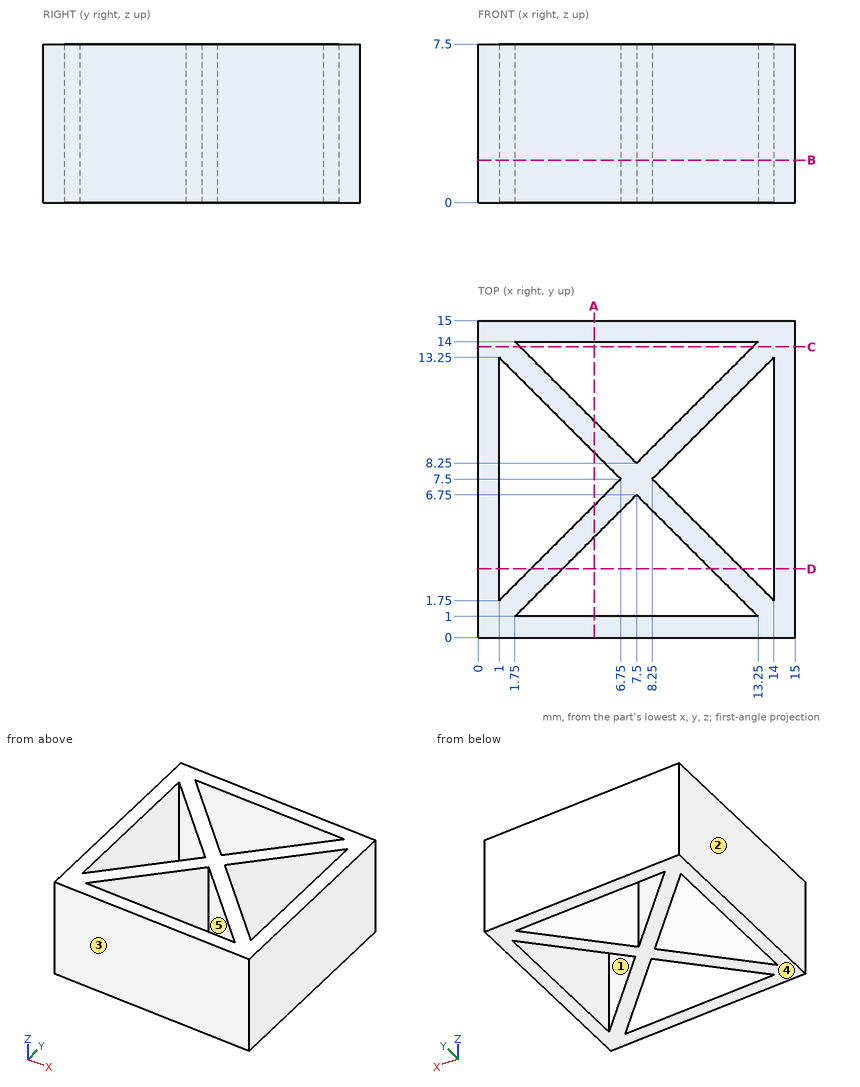
Answer from the drawing. Dimensions are ordinates in mm from the lowest x, y and z of the part. A direction names the side the tool comes from. Coordinates: 2 decimals unless noted, no trailing zeros. Order: outer loops, then holes, each group sorted by start corner. A loop starts at its lowest first (then second) coordinate and runs counter-clockwise, first axis right, second up. Notation, with made-up numbers: (-15.75, 52) - (5.25, 52) arc R14 cw to (5.25, 76) - close; hole circle Ø2 at (8.25, 61). An arc over 180 degrees is marked (long way). Use one line per item in the form item = value.
(1) Section D-D, the plane y = 3.25 is taken. Give the vertices of the cut face in (x, z).
Computed values:
outline = (0, 0) - (1, 0) - (1, 7.5) - (0, 7.5) - close; (2.5, 0) - (4, 0) - (4, 7.5) - (2.5, 7.5) - close; (11, 0) - (12.5, 0) - (12.5, 7.5) - (11, 7.5) - close; (14, 0) - (15, 0) - (15, 7.5) - (14, 7.5) - close
(2) Straight lines are drawn through the part: L1, parallel to Y at x = 10.75, z = 4.5; L2, parallel to X at y = 5.5, z = 2.5; L3, parallel to X at y = 8.5, z = 0.5. For each, find the intervals that lie inside material, in ascending order.
Computed values:
L1 = 0 to 1, 3.5 to 5, 10 to 11.5, 14 to 15
L2 = 0 to 1, 4.75 to 6.25, 8.75 to 10.25, 14 to 15
L3 = 0 to 1, 5.75 to 7.25, 7.75 to 9.25, 14 to 15
(3) For a pull along X with two mould halves and no side action, classify the marked faces 1, 2 and 3 as pulls with the +X half, pulls with the -X half, needs draft (parallel to the pull), parting line crosses it, or undercut.
Computed values:
face_1 = undercut
face_2 = pulls with the -X half
face_3 = needs draft
(4) Section C-C, the plane y = 13.75 is taken. Give the vertices of the cut face in (x, z), then the cut area to 3 significant figures.
Computed values:
outline = (0, 0) - (2, 0) - (2, 7.5) - (0, 7.5) - close; (13, 0) - (15, 0) - (15, 7.5) - (13, 7.5) - close
area = 30.0 mm²
(5) Section B-B, the plane z = 2 is taken. Give the vertices of the cut face in (x, y), then the cut area to 4 significant figures.
Computed values:
outline = (0, 0) - (15, 0) - (15, 15) - (0, 15) - close; hole (1, 1.75) - (6.75, 7.5) - (1, 13.25) - close; hole (1.75, 1) - (13.25, 1) - (7.5, 6.75) - close; hole (1.75, 14) - (7.5, 8.25) - (13.25, 14) - close; hole (8.25, 7.5) - (14, 1.75) - (14, 13.25) - close
area = 92.75 mm²
(6) Which of the six approach directions +Z, -Z, +X, -X, +Y, -Y give full straight-line access (tool end or side, diameter ignored) to the marked faces 4 and 5?
Computed values:
face_4 = -Z, +X, -X, +Y, -Y
face_5 = +Z, -Z
(7) Section A-A, the plane x = 5.5 is taken. Give the vertices of the cut face in (y, z).
Computed values:
outline = (0, 0) - (1, 0) - (1, 7.5) - (0, 7.5) - close; (4.75, 0) - (6.25, 0) - (6.25, 7.5) - (4.75, 7.5) - close; (8.75, 0) - (10.25, 0) - (10.25, 7.5) - (8.75, 7.5) - close; (14, 0) - (15, 0) - (15, 7.5) - (14, 7.5) - close
